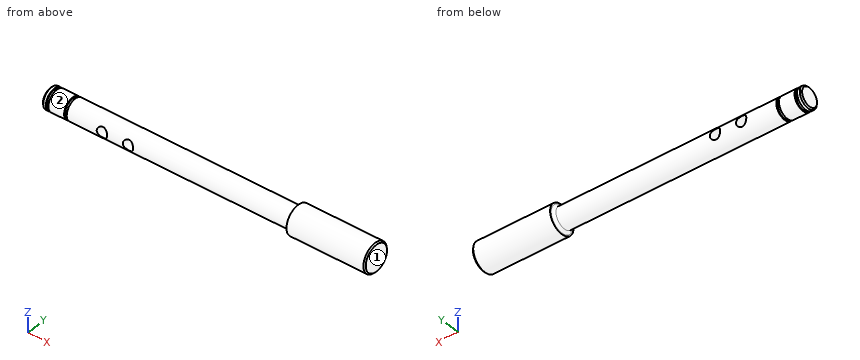
```python
from build123d import *

# Parameters (mm, degrees)
CUT_EXTRUDE_1_DEPTH      = 10
CUT_EXTRUDE_1_DEPTH_BACK = 10
SKETCH_2_R               = 2


with BuildPart() as part:
    # Sketch 1 → Revolve 1 (revolve)
    with BuildSketch(Plane.XY, mode=Mode.PRIVATE) as revolve_1_sk:
        with BuildLine():
            Line((-32.999870063, 0), (-32.999870063, 3.5))
            Line((-32.999870063, 3.5), (-32.499870063, 4))
            Line((-32.499870063, 4), (-31.499870063, 4))
            Line((-31.499870063, 4), (-31.499870063, 3.5))
            Line((-31.499870063, 3.5), (-30.499870063, 3.5))
            Line((-30.499870063, 3.5), (-30.499870063, 4))
            Line((-30.499870063, 4), (-24.499870063, 4))
            Line((-24.499870063, 4), (-24.499870063, 3.5))
            Line((-24.499870063, 3.5), (-23.499870063, 3.5))
            Line((-23.499870063, 3.5), (-23.499870063, 4))
            Line((-23.499870063, 4), (61, 4))
            ThreePointArc((61, 4), (61.707106781, 4.292893219), (62, 5))
            Line((62, 5), (62, 5.5))
            Line((62, 5.5), (91.5, 5.5))
            Line((91.5, 5.5), (92, 5))
            Line((92, 5), (92, 0))
            Line((92, 0), (-32.999870063, 0))
        make_face()
    revolve(revolve_1_sk.sketch.rotate(Axis((-32.999870063, 0, 0), (1, 0, 0)), 180), axis=Axis((-32.999870063, 0, 0), (1, 0, 0)))

    # Sketch 2 → Cut-Extrude 1 (cut, two sides: drawn at the far end of the back side and taken through both)
    with BuildSketch(Plane(origin=(0, 0, 0), x_dir=(1, 0, 0), z_dir=(0, 1, 0)).offset(-CUT_EXTRUDE_1_DEPTH_BACK)):
        with Locations(Location((-9.999870063, 0, 0), (0, 0, 90))):
            Circle(SKETCH_2_R)
        with Locations(Location((0.000129937, 0, 0), (0, 0, 90))):
            Circle(SKETCH_2_R)
    extrude(amount=CUT_EXTRUDE_1_DEPTH + CUT_EXTRUDE_1_DEPTH_BACK, mode=Mode.SUBTRACT)


solid = part.part
```
Input: part model. Units: mm. Frame: model coordinates. Face numbers are marked on the shaded views. A direction names the side the tool comes from. Coordinates: 2 decimals unless noted, no trailing zeros. Loops run counter-clockwise (first coordinate to the right, second up) from the corner with the lowest first, then second, coordinate; pieces in that order, holes last. Notation, with made-up numbers: M -20.5,56 L 16.5,56 A14 ccw 16.5,63 Z; hole C 87,29.25 d5. An arc over 180 degrees is marked long. Use a Markdown table: item, result. Add a question column.
1) Section A-A, the plane z = 0. Give the number of separate pieces and of enclosed holes in the cut face, plus the area to 3 significant figures.
2) Line query: L1, parallel to X at y = 0.5, z = 0; L2, parallel to X at y = -3, z = 1.5; L3, parallel to X at y = -3.5, z = 1.5. Output: solid intervals per line, ascending. Write a range as from..to.
3) Section B-B, the plane x = -20.5. Return the cut outline in (y, z).
4) Set-up query: the marked faces 1 and 2. Return all of +Z, -Z, +X, -X, +Y, -Y with unobstructed straight access to the full face (end or side cutting, diameter ignored); none if empty.
5) Pin query (flat end, axial travel): P1, Ø3.5, axis at x = -10, z = 0, coming from the +Y side; P2, Ø2, axis at x = -13.5, z = 4.5, coming from the +Y side; P3, Ø4, axis at x = 64, y = 0.5, coming from the +Z side; P4, Ø3, axis at x = 56, z = 2, coming from the +Y side. Return the tip coordinate at first contact, or that it passes through.
Answer below:
| question | item | result |
|---|---|---|
| 1 | separate pieces | 3 |
| 1 | enclosed holes | 0 |
| 1 | area | 1,020 mm2 |
| 2 | L1 | -33..-12, -8..-2, 2..92 |
| 2 | L2 | -33..-11.32, -8.68..-1.32, 1.32..92 |
| 2 | L3 | -32.69..-31.5, -30.5..-24.5, -23.5..-11.32, -8.68..-1.32, 1.32..92 |
| 3 | outline | C 0,0 d8 |
| 4 | face 1 | +Z, -Z, +X, +Y, -Y |
| 4 | face 2 | -X |
| 5 | P1 | through |
| 5 | P2 | y = 1.94 |
| 5 | P3 | z = 5.5 |
| 5 | P4 | y = 3.97 |
